Autodesk Inventor part; units mm, degrees
ref_plane "YZ Plane" through (0, 0, 0) normal (1, 0, 0) x (0, 1, 0)
ref_plane "XZ Plane" through (0, 0, 0) normal (0, 1, 0) x (-1, 0, 0)
ref_plane "XY Plane" through (0, 0, 0) normal (0, 0, 1) x (1, 0, 0)
sketch "Sketch1" plane through (0, 0, 0) normal (1, 0, 0) x (0, 1, 0)
  circle A0 centre (0, 0) radius 188.9
  circle A1 centre (0, 0) radius 163.9
  dimension "d0" = 377.8
  dimension "d2" = 327.8
extrude "Extrusion1" add sketch "Sketch1" along normal blind 15
sketch "Sketch2" plane through (15, 0, 0) normal (1, 0, 0) x (0, 0, -1)
  circle A0 centre (0, 0) radius 176.5
  circle A1 centre (0, 176.5) radius 5
  dimension "d5" = 353
  dimension "d6" = 10
extrude "Extrusion2" cut sketch "Sketch2" against normal through all contours A1 A0 | A0 A1 picked at (0.1991, 174.84) picked at (0.1901, 178.1505)
pattern_circular "Circular Pattern1" count 8 over 360 about axis through (0, 0, 0) along (1, 0, 0) of "Extrusion2"
sketch "Sketch3" plane through (0, 0, 0) normal (-1, 0, 0) x (0, 0, 1)
  circle A0 centre (0, 0) radius 163.9
  circle A1 centre (0, 0) radius 158.9
  dimension "d12" = 317.8
extrude "Extrusion3" add sketch "Sketch3" against normal blind 40
sketch "Sketch4" plane through (0, 0, 0) normal (0, 0, 1) x (1, 0, 0)
  line L0 (40, 158.9) -> (40, -158.9)
  line L1 (40, -163.9) -> (40, 163.9)
  line L2 (30, 153.9) -> (30, 158.9)
  line L3 (30, 158.9) -> (40, 158.9)
  line L4 (40, 158.9) -> (40, 153.9)
  line L5 (30, 153.9) -> (30, 134)
  line L6 (40, 134) -> (40, 153.9)
  line L7 (-8, 0) -> (48, 0)
  line L8 (40, 158.9) -> (40, 134)
  line L9 (30, 134) -> (20, 134)
  line L10 (20, 134) -> (20, 131)
  line L11 (20, 131) -> (30, 131)
  line L12 (30, 131) -> (30, 126)
  line L13 (30, 126) -> (20, 126)
  line L14 (20, 126) -> (20, 123)
  line L15 (20, 123) -> (30, 123)
  line L16 (30, 123) -> (30, 118)
  line L17 (30, 118) -> (20, 118)
  line L18 (20, 118) -> (20, 115)
  line L19 (20, 115) -> (40, 115)
  line L20 (40, 115) -> (40, 134)
  point P0 (0, 0)
revolve "Revolution1" add sketch "Sketch4" angle 360 about axis through (-10, 0, 0) along (1, 0, 0)
thread "Thread1"
thread "Thread2"
thread "Thread3"
thread "Thread4"
thread "Thread5"
thread "Thread6"
thread "Thread7"
thread "Thread8"
properties part number "lavyrintosecondchance"
The model under review builds one solid part; all positions refer to its coordinate system, in mm. A direction names the side the tool comes from. Round coordinates to 2 decimals unless told otherwise and drop trailing zeros. Write each loop counter-clockwise with the first axis right and the second up, starting at its lowest first coordinate (ties: lowest second). Pieces come first, ordered by that corner, then holes. Notation, with made-up numbers: M 79.25,39.5 L 111.25,39.5 A31 ccw 111.25,77.5 Z; hole C 18,26 d9. An arc over 180 degrees is marked long. Answer as CSV lines item,"result". Start each with the question number.
Q1. The part is to be moulded in two halves that separate along Y. For faces 4 (the face through (27.32, 49.23, 156.33)), 5 (the face through (0, -99, 127)), 6 (the face through (30.14, -24.93, -112.265)), say which applies: +Y half, -Y half, draft (parallel to the pull), parting line (faces both ways), or undercut.
Q2. Clearance check with flat-ended pins moving along their axes: P1, Ø6, axis at x = 19, y = -123.5, coming from the +Z side; P2, Ø4, axis at x = 10.5, z = 27, coming from the -Y side; P3, Ø12, axis at x = 30.5, y = -39, coming from the -Z side. State where each tip first meets the part, or that it passes through.
Q3. Consider section A-A, the plane z = 176.5. Give the boundary of the cut face in (x, y), then the cut area to 3 significant figures.
Q4. Wall thickness on line 1 along Z through (x, y) = (8.5, 0); line 2 along X through (y, z) = (98, 82); line 3 along Z through (x, y) = (34, 0): over which ranges is each line inside the solid? List them lowest first.
Q5. Tool access review of faces 1 (the face through (7.605, -0.651, 181.457)), 2 (the face through (24.93, 112.551, -35.444)), 3 (the face through (15, -57, 155)): name each direction out of +Z, -Z, +X, -X, +Y, -Y from which nothing blocks a thin tool from reaching the whole face with its end or side.
Q6. Consider section B-B, the plane y = 0. State how many separate pieces and enclosed holes the cut face has, then the cut area to 3 significant figures.
Result set:
1,face 4,"parting line"
1,face 5,"draft"
1,face 6,"undercut"
2,P1,"stops at z = 111.1"
2,P2,"stops at y = -187.24"
2,P3,"stops at z = -160.54"
3,outline,"M 0,-67.31 L 15,-67.31 L 15,-5 L 0,-5 Z; M 0,5 L 15,5 L 15,67.31 L 0,67.31 Z"
3,area,"1,870 mm²"
4,line 1,"z = -188.9 to -181.5, -171.5 to -158.9, 158.9 to 171.5, 181.5 to 188.9"
4,line 2,"x = 30 to 40"
4,line 3,"z = -163.9 to -115, 115 to 163.9"
5,face 1,"+X, -X"
5,face 2,"-X"
5,face 3,"+X"
6,separate pieces,"4"
6,enclosed holes,"0"
6,area,"1,910 mm²"
